Design review of the part built by this model. Coordinates are the model's own, in mm. Round coordinates to 2 decimals unless told otherwise and drop trailing zeros. Order: outer loops, then holes, each group sorted by start corner. A loop starts at its lowest first (then second) coordinate and runs counter-clockwise, first axis right, second up. Notation, with made-up numbers: M 27,65.25 L 46,65.25 A11 ccw 46,70.25 Z; hole C 24.5,58.25 d4. An arc over 180 degrees is marked long. Use a Markdown table: item, result. Add a question column.
(1) Take a section at C-C (x = -17.5). Write out the cut boundary in (y, z), then the cut area to 3 significant figures.
(2) Take a section at B-B (z = 9.5). Write out the cut boundary in (x, y), then the cut area to 3 significant figures.
(3) To check wall thickness, follow probe 1 along X at (y, z) = (-63, 5); probe 2 along X at (y, z) = (-255, 2.5); probe 3 along Y at (x, z) = (-29, 20). State the ranges of each line that lie inside material, in increasing order. Write a range as from..to.
(4) Take a section at A-A (y = -195.5). Write out the cut boundary in (x, z), then the cut area to 3 significant figures.
(5) For pin 1 (3 mm diameter, centred on x = -6.5, y = -151, fed in from -Z); pin 2 (5 mm diameter, centred on y = -61, z = 7, fed in from +X); pin 3 (1 mm diameter, centred on x = -12.5, y = -157.5, fed in from -Z), all flat-tipped, find the tip position at first contact; note any pin that passes through.
```python
from build123d import *

# Parameters (mm, degrees)
F1_DEPTH = 285.75
F3_DEPTH = 50.8


with BuildPart() as f1:
    # F0 (on Front) → F1 (new body)
    with BuildSketch(Plane.XZ):
        with BuildLine():
            Line((-31.75, 0), (-25.4, 0))
            ThreePointArc((-25.4, 0), (-17.960512, 17.960512), (0, 25.4))
            Line((0, 25.4), (0, 31.75))
            Line((0, 31.75), (-31.75, 31.75))
            Line((-31.75, 31.75), (-31.75, 0))
        make_face()
    extrude(amount=F1_DEPTH)

    # F2 (on face) → F3 (cut)
    with BuildSketch(Plane.XY.offset(31.75)):
        Polygon((-31.75, -285.75), (0, -285.75), (-31.75, -254), align=None)
    extrude(amount=-F3_DEPTH, mode=Mode.SUBTRACT)


solid = f1.part
```
Verdict:
| question | item | result |
|---|---|---|
| 1 | outline | M -268.25,18.41 L 0,18.41 L 0,31.75 L -268.25,31.75 Z |
| 1 | area | 3,580 mm^2 |
| 2 | outline | M -31.75,-254 L -23.56,-262.19 L -23.56,0 L -31.75,0 Z |
| 2 | area | 2,110 mm^2 |
| 3 | probe 1 | x = -31.75..-24.9 |
| 3 | probe 2 | x = -30.75..-25.28 |
| 3 | probe 3 | y = -256.75..0 |
| 4 | outline | M -31.75,0 L -25.4,0 A25.4 cw 0,25.4 L 0,31.75 L -31.75,31.75 Z |
| 4 | area | 501 mm^2 |
| 5 | pin 1 | stops at z = 24.11 |
| 5 | pin 2 | stops at x = -23.56 |
| 5 | pin 3 | stops at z = 21.82 |
